Here's how the part is built. I have some questions about the finished solid (model axes, mm). A direction names the side the tool comes from. Round coordinates to 2 decimals unless told otherwise and drop trailing zeros. Loops run counter-clockwise (first coordinate to the right, second up) from the corner with the lowest first, then second, coordinate; pieces in that order, holes last. Notation, with made-up numbers: M 79,28 L 89,28 A21 cw 89,57 Z; hole C 46,-9.5 d3. An arc over 180 degrees is marked long. Use a Markdown table: item, result.
from build123d import *

# Parameters (mm, degrees)
SKETCH1_W                  = 85
SKETCH1_H                  = 128
TOP_LID_DEPTH              = 6
SKETCH2_R                  = 1.75
SCREW_HOLE_DEPTH           = 10
SKETCH5_R                  = 2.5
SCREW_HEAD_DEPTH           = 2
SCREW_HEAD_DRAFT           = -45
SCREW_HEAD_PROFILE_2_DEPTH = 2
SCREW_HEAD_PROFILE_2_DRAFT = -45
SCREW_HEAD_PROFILE_3_DEPTH = 2
SCREW_HEAD_PROFILE_3_DRAFT = -45
SCREW_HEAD_PROFILE_4_DEPTH = 2
SCREW_HEAD_PROFILE_4_DRAFT = -45
SCREW_HEAD_PROFILE_5_DEPTH = 2
SCREW_HEAD_PROFILE_5_DRAFT = -45
SKETCH6_W                  = 71
SKETCH6_H                  = 121
DEVICE_CUT_OUT_DEPTH       = 2.25
SKETCH7_W                  = 10
SKETCH7_H                  = 40
SLIDERS_DEPTH              = 4
FILLET1_R                  = 2
FILLET2_R                  = 2
FILLET3_R                  = 2
FILLET4_R                  = 2


with BuildPart() as part:
    # Sketch1 → Top Lid (new body)
    with BuildSketch(Plane(origin=(0, 0, 0), x_dir=(1, 0, 0), z_dir=(0, 1, 0))):
        Rectangle(SKETCH1_W, SKETCH1_H)
    extrude(amount=TOP_LID_DEPTH)

    # Sketch2 → Screw Hole (cut)
    with BuildSketch(Plane.XZ):
        with Locations(Location((39, 59, 0), (0, 0, 270))):
            Circle(SKETCH2_R)
        with Locations(Location((-39, 59, 0), (0, 0, 270))):
            Circle(SKETCH2_R)
        with Locations(Location((-39, 1.83, 0), (0, 0, 270))):
            Circle(SKETCH2_R)
        with Locations(Location((39, 1.83, 0), (0, 0, 270))):
            Circle(SKETCH2_R)
        with Locations(Location((0, -60.5, 0), (0, 0, 270))):
            Circle(SKETCH2_R)
    extrude(amount=-SCREW_HOLE_DEPTH, mode=Mode.SUBTRACT)


with BuildPart() as screw_head_tool:
    # Sketch5 → Screw Head (with draft: the straight prism first)
    with BuildSketch(Plane.XZ):
        with Locations((39, 59)):
            Circle(SKETCH5_R)
    extrude(amount=-SCREW_HEAD_DEPTH)
    # Screw Head: the draft: its side faces are tilted about the plane it starts from
    screw_head_sides = [screw_head_tool.faces().sort_by_distance(p)[0] for p in [
        (36.5, 1, 59),
    ]]
    draft(screw_head_sides, Plane.XZ, SCREW_HEAD_DRAFT)


with BuildPart() as part_1:
    add(part.part)

    # Screw Head: cut by screw_head_tool
    add(screw_head_tool.part, mode=Mode.SUBTRACT)


with BuildPart() as screw_head_profile_2_tool:
    # Sketch5 → Screw Head profile 2 (with draft: the straight prism first)
    with BuildSketch(Plane.XZ):
        with Locations((-39, 59)):
            Circle(SKETCH5_R)
    extrude(amount=-SCREW_HEAD_PROFILE_2_DEPTH)
    # Screw Head profile 2: the draft: its side faces are tilted about the plane it starts from
    screw_head_profile_2_sides = [screw_head_profile_2_tool.faces().sort_by_distance(p)[0] for p in [
        (-41.5, 1, 59),
    ]]
    draft(screw_head_profile_2_sides, Plane.XZ, SCREW_HEAD_PROFILE_2_DRAFT)


with BuildPart() as part_2:
    add(part_1.part)

    # Screw Head profile 2: cut by screw_head_profile_2_tool
    add(screw_head_profile_2_tool.part, mode=Mode.SUBTRACT)


with BuildPart() as screw_head_profile_3_tool:
    # Sketch5 → Screw Head profile 3 (with draft: the straight prism first)
    with BuildSketch(Plane.XZ):
        with Locations((-39, 1.83)):
            Circle(SKETCH5_R)
    extrude(amount=-SCREW_HEAD_PROFILE_3_DEPTH)
    # Screw Head profile 3: the draft: its side faces are tilted about the plane it starts from
    screw_head_profile_3_sides = [screw_head_profile_3_tool.faces().sort_by_distance(p)[0] for p in [
        (-41.5, 1, 1.83),
    ]]
    draft(screw_head_profile_3_sides, Plane.XZ, SCREW_HEAD_PROFILE_3_DRAFT)


with BuildPart() as part_3:
    add(part_2.part)

    # Screw Head profile 3: cut by screw_head_profile_3_tool
    add(screw_head_profile_3_tool.part, mode=Mode.SUBTRACT)


with BuildPart() as screw_head_profile_4_tool:
    # Sketch5 → Screw Head profile 4 (with draft: the straight prism first)
    with BuildSketch(Plane.XZ):
        with Locations((39, 1.83)):
            Circle(SKETCH5_R)
    extrude(amount=-SCREW_HEAD_PROFILE_4_DEPTH)
    # Screw Head profile 4: the draft: its side faces are tilted about the plane it starts from
    screw_head_profile_4_sides = [screw_head_profile_4_tool.faces().sort_by_distance(p)[0] for p in [
        (36.5, 1, 1.83),
    ]]
    draft(screw_head_profile_4_sides, Plane.XZ, SCREW_HEAD_PROFILE_4_DRAFT)


with BuildPart() as part_4:
    add(part_3.part)

    # Screw Head profile 4: cut by screw_head_profile_4_tool
    add(screw_head_profile_4_tool.part, mode=Mode.SUBTRACT)


with BuildPart() as screw_head_profile_5_tool:
    # Sketch5 → Screw Head profile 5 (with draft: the straight prism first)
    with BuildSketch(Plane.XZ):
        with Locations((0, -60.5)):
            Circle(SKETCH5_R)
    extrude(amount=-SCREW_HEAD_PROFILE_5_DEPTH)
    # Screw Head profile 5: the draft: its side faces are tilted about the plane it starts from
    screw_head_profile_5_sides = [screw_head_profile_5_tool.faces().sort_by_distance(p)[0] for p in [
        (-2.5, 1, -60.5),
    ]]
    draft(screw_head_profile_5_sides, Plane.XZ, SCREW_HEAD_PROFILE_5_DRAFT)


with BuildPart() as part_5:
    add(part_4.part)

    # Screw Head profile 5: cut by screw_head_profile_5_tool
    add(screw_head_profile_5_tool.part, mode=Mode.SUBTRACT)

    # Sketch6 → Device cut out (cut)
    with BuildSketch(Plane(origin=(0, 6, 0), x_dir=(1, 0, 0), z_dir=(0, 1, 0))):
        with Locations((0, -3.5)):
            Rectangle(SKETCH6_W, SKETCH6_H)
    extrude(amount=-DEVICE_CUT_OUT_DEPTH, mode=Mode.SUBTRACT)

    # Sketch7 → Sliders (cut)
    with BuildSketch(Plane(origin=(0, 6, 0), x_dir=(1, 0, 0), z_dir=(0, 1, 0))):
        with Locations((34.5, -34)):
            Rectangle(SKETCH7_W, SKETCH7_H)
        with Locations((-34.5, -34)):
            Rectangle(SKETCH7_W, SKETCH7_H)
    extrude(amount=-SLIDERS_DEPTH, mode=Mode.SUBTRACT)

    # Fillet1
    fillet1_edges = [part_5.edges().sort_by_distance(p)[0] for p in [
        (42.5, 3, 64),
    ]]
    fillet(fillet1_edges, radius=FILLET1_R)

    # Fillet2
    fillet2_edges = [part_5.edges().sort_by_distance(p)[0] for p in [
        (42.5, 3, -64),
    ]]
    fillet(fillet2_edges, radius=FILLET2_R)

    # Fillet3
    fillet3_edges = [part_5.edges().sort_by_distance(p)[0] for p in [
        (-42.5, 3, -64),
    ]]
    fillet(fillet3_edges, radius=FILLET3_R)

    # Fillet4
    fillet4_edges = [part_5.edges().sort_by_distance(p)[0] for p in [
        (-42.5, 3, 64),
    ]]
    fillet(fillet4_edges, radius=FILLET4_R)


solid = part_5.part
1. We'd pull the mould along X, two halves only. Please class faces 3 (the face through (37.29, 3.34, 2.21)), 4 (the face through (42.5, 3, 1)), 5 (the face through (-1, 2, 64)), 6 (the face through (-42.5, 3, 1)): +X half, -X half, draft (parallel to the pull), parting line (faces both ways), or undercut.
Answer sheet:
| item | result |
|---|---|
| face 3 | undercut |
| face 4 | +X half |
| face 5 | draft |
| face 6 | -X half |
2. Imagine slicing it at A-A, the plane z = -60.5. Write out the boundary of the cut face in (x, y), then the cut area to 3 significant figures.
Answer sheet:
| item | result |
|---|---|
| outline | M -42.5,0 L -2.5,0 L -1.75,0.75 L -1.75,6 L -42.5,6 Z; M 1.75,0.75 L 2.5,0 L 42.5,0 L 42.5,6 L 1.75,6 Z |
| area | 488 mm2 |
3. Which directions (+Z, -Z, +X, -X, +Y, -Y) give clear straight access to the entire face, cutting with the end or side of a thin tool? Please do faces 1 (the face through (-40.71, 3.34, 2.21)), 2 (the face through (36, 4, 14)).
Answer sheet:
| item | result |
|---|---|
| face 1 | +Y, -Y |
| face 2 | +Y |
4. Imagine slicing it at B-B, the plane x = 0. Write out the boundary of the cut face in (y, z), then the cut area to 3 significant figures.
Answer sheet:
| item | result |
|---|---|
| outline | M 0,-64 L 6,-64 L 6,-62.25 L 0.75,-62.25 L 0,-63 Z; M 0,-58 L 0.75,-58.75 L 6,-58.75 L 6,-57 L 3.75,-57 L 3.75,64 L 0,64 Z |
| area | 474 mm2 |
5. For pin 1 Ø11 at (x, z) = (33.5, 30.5) entering from +Y; pin 2 Ø3 at (x, z) = (39, 59) entering from -Y, each with a flat end and sliding along its axis, tell me the tip position at first contact or that it passes through.
Answer sheet:
| item | result |
|---|---|
| pin 1 | y = 3.75 |
| pin 2 | through |
6. I need wall thicknesses on probe 1 along Z at (x, y) = (39, 2.4); probe 2 along X at (y, z) = (2.1, 22); probe 3 along X at (y, z) = (4.05, 59). Which ranges of each line are inside material? Lowest first, please. Write a range as from..to.
Answer sheet:
| item | result |
|---|---|
| probe 1 | -64..0.08, 3.58..14, 54..57.25, 60.75..64 |
| probe 2 | -42.5..-39.5, -29.5..29.5, 39.5..42.5 |
| probe 3 | -42.5..-40.75, -37.25..-35.5, 35.5..37.25, 40.75..42.5 |
7. Imagine slicing it at C-C, the plane y = 4.75. Write out the boundary of the cut face in (x, z), then the cut area to 3 significant figures.
Answer sheet:
| item | result |
|---|---|
| outline | M -42.5,-62 A2 ccw -40.5,-64 L 40.5,-64 A2 ccw 42.5,-62 L 42.5,62 A2 ccw 40.5,64 L 35.5,64 L 35.5,54 L 39.5,54 L 39.5,14 L 35.5,14 L 35.5,-57 L -35.5,-57 L -35.5,14 L -39.5,14 L -39.5,54 L -35.5,54 L -35.5,64 L -40.5,64 A2 ccw -42.5,62 Z; hole C -39,1.83 d3.5; hole C -39,59 d3.5; hole C 0,-60.5 d3.5; hole C 39,1.83 d3.5; hole C 39,59 d3.5 |
| area | 1,920 mm2 |
8. Imagine slicing it at D-D, the plane z = 1.83. Write out the boundary of the cut face in (x, y).
Answer sheet:
| item | result |
|---|---|
| outline | M -42.5,0 L -41.5,0 L -40.75,0.75 L -40.75,6 L -42.5,6 Z; M -37.25,0.75 L -36.5,0 L 36.5,0 L 37.25,0.75 L 37.25,6 L 35.5,6 L 35.5,3.75 L -35.5,3.75 L -35.5,6 L -37.25,6 Z; M 40.75,0.75 L 41.5,0 L 42.5,0 L 42.5,6 L 40.75,6 Z |
